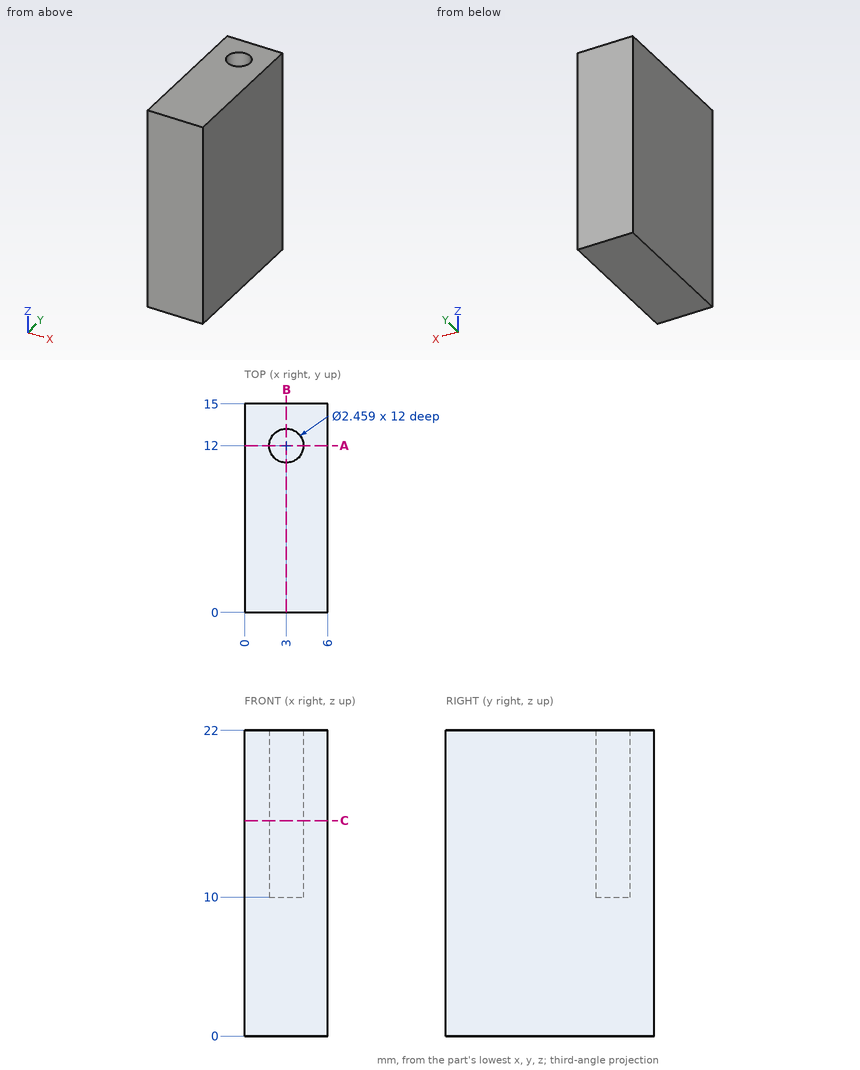
The drawing under review shows one solid part. Ordinate dimensions are in mm from its lowest x, y, z. Coordinates: 2 decimals unless noted, no trailing zeros. Loops run counter-clockwise (first coordinate to the right, second up) from the corner with the lowest first, then second, coordinate; pieces in that order, holes last.
Item 1: Clearance check with flat-ended pins moving along their axes: pin 1 (5 mm diameter, centred on y = 2.5, z = 2.5, fed in from -X); pin 2 (0.7 mm diameter, centred on x = 2.5, y = 12, fed in from +Z). State where each tip first meets the part, or that it passes through.
Completed:
pin 1: stops at x = 0
pin 2: stops at z = 10
Item 2: Add section C-C (z = 15.5). Write out the cut boundary in (x, y), and give its area (3 significant figures).
Completed:
outline: (0, 0) - (6, 0) - (6, 15) - (0, 15) - close; hole circle Ø2.46 at (3, 12)
area: 85.3 mm2
Item 3: Add section A-A (y = 12). Write out the cut boundary in (x, z), and give its area (3 significant figures).
Completed:
outline: (0, 0) - (6, 0) - (6, 22) - (4.23, 22) - (4.23, 10) - (1.77, 10) - (1.77, 22) - (0, 22) - close
area: 102 mm2
Item 4: Wall thickness on L1, parallel to X at y = 12, z = 13.25; L2, parallel to Y at x = 3, z = 16.5; L3, parallel to Y at x = 4, z = 18.75: over which ranges is each line inside the solid? List them lowest first.
Completed:
L1: x = 0 to 1.77, 4.23 to 6
L2: y = 0 to 10.77, 13.23 to 15
L3: y = 0 to 11.28, 12.72 to 15
Item 5: Add section B-B (x = 3). Write out the cut boundary in (y, z).
Completed:
outline: (0, 0) - (15, 0) - (15, 22) - (13.23, 22) - (13.23, 10) - (10.77, 10) - (10.77, 22) - (0, 22) - close
